Could you check a few things on this model? Use its own coordinates, in mm. Give positions to 0.01 mm unless a question says otherwise; leave off trailing zeros. Write each loop counter-clockwise with the first axis right and the second up, starting at its lowest first coordinate (ties: lowest second). Pieces come first, ordered by that corner, then holes. Notation, with made-up numbers: (57.25, 31.5) - (99.25, 31.5) arc R23 cw to (99.25, 39.5) - close; hole circle Ø8 at (58, 45). An arc over 180 degrees is marked (long way). Use one line per item in the form item = value.
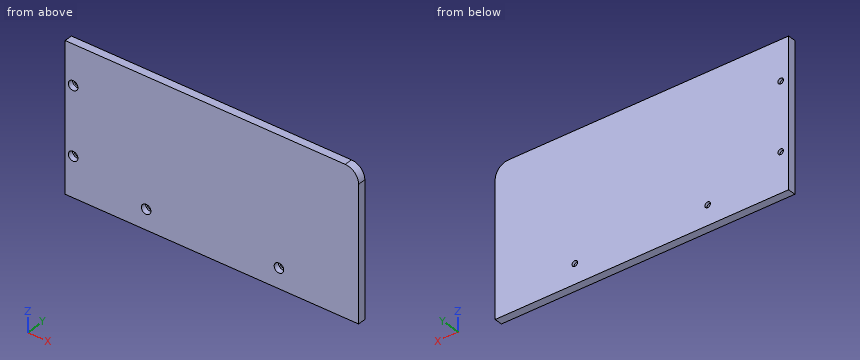
Autodesk Inventor part; units mm, degrees
ref_plane "YZ Plane" through (0, 0, 0) normal (1, 0, 0) x (0, 1, 0)
ref_plane "XZ Plane" through (0, 0, 0) normal (0, 1, 0) x (-1, 0, 0)
ref_plane "XY Plane" through (0, 0, 0) normal (0, 0, 1) x (1, 0, 0)
sketch "草图1" plane through (0, 0, 0) normal (0, 1, 0) x (-1, 0, 0)
  line L0 (110.5, 55.5) -> (-110.5, 55.5)
  line L1 (-110.5, 55.5) -> (-110.5, -55.5)
  line L2 (-110.5, -55.5) -> (110.5, -55.5)
  line L3 (110.5, -55.5) -> (110.5, 55.5)
  line L4 (0, 7.5575) -> (0, -11)
  line L5 (8.5019, 0) -> (-7, 0)
  point P0 (0, 0)
  point P1 (0, 0)
  dimension "d0" = 221
  dimension "d1" = 111
extrude "拉伸1" add sketch "草图1" along normal blind 6
fillet "圆角1" radius 10.1 1 edges at (110.5, 3, 55.5)
sketch "草图2" plane through (0, 0, 0) normal (0, -1, 0) x (1, 0, 0)
  circle A0 centre (-104.5, 25.5) radius 2.1
  circle A1 centre (-104.5, -25.5) radius 2.1
  line L0 (-110.5, -55.5) -> (-110.5, 55.5)
  line L1 (110.5, -55.5) -> (-110.5, -55.5)
  line L2 (-110.5, 55.5) -> (100.4, 55.5)
  point P0 (0, 0)
  dimension "d5" = 4.2
  dimension "d6" = 4.2
  dimension "d7" = 6
  dimension "d8" = 6
  dimension "d9" = 30
  dimension "d10" = 30
extrude "拉伸2" cut sketch "草图2" against normal blind 6
sketch "草图3" plane through (0, 0, 0) normal (0, -1, 0) x (1, 0, 0)
  circle A0 centre (-104.5, 25.5) radius 2.1
  circle A1 centre (-104.5, 25.5) radius 3.6
  circle A2 centre (-104.5, -25.5) radius 2.1
  circle A3 centre (-104.5, -25.5) radius 3.6
  point P0 (0, 0)
  dimension "d13" = 7.2
  dimension "d14" = 7.2
extrude "拉伸3" cut sketch "草图3" against normal blind 4
sketch "草图4" plane through (0, 0, 0) normal (0, -1, 0) x (1, 0, 0)
  circle A0 centre (-49.5, -40.5) radius 2.1
  circle A1 centre (50.5, -40.5) radius 2.1
  line L0 (110.5, -55.5) -> (-110.5, -55.5)
  line L1 (110.5, 45.4) -> (110.5, -55.5)
  point P0 (0, 0)
  dimension "d17" = 4.2
  dimension "d18" = 4.2
  dimension "d19" = 15
  dimension "d20" = 15
  dimension "d21" = 60
  dimension "d22" = 100
extrude "拉伸4" cut sketch "草图4" against normal blind 10
sketch "草图5" plane through (0, 0, 0) normal (0, -1, 0) x (1, 0, 0)
  circle A0 centre (-49.5, -40.5) radius 2.1
  circle A1 centre (-49.5, -40.5) radius 3.6
  circle A2 centre (50.5, -40.5) radius 2.1
  circle A3 centre (50.5, -40.5) radius 3.6
  point P0 (0, 0)
  dimension "d25" = 7.2
  dimension "d26" = 7.2
extrude "拉伸5" cut sketch "草图5" against normal blind 4 contours A0 | A1 | A2 | A3
properties part number "底板_B"
1. If I drill on line 1 (Z direction, x = -49.5, y = 5.4); line 2 (X direction, y = 3.1, z = 24), over which ranges is the centre line in solid material (lowest first)? Write a range as from..to.
Response values:
line_1 = -55.5..-42.6, -38.4..55.5
line_2 = -110.5..-107.77, -101.23..110.5
2. Imagine slicing it at B-B, the plane z = 25.5. List the corners of the cut face in (x, y) for me, and give its area (3 significant figures).
Response values:
outline = (-110.5, 0) - (-108.1, 0) - (-108.1, 4) - (-106.6, 4) - (-106.6, 6) - (-110.5, 6) - close; (-102.4, 4) - (-100.9, 4) - (-100.9, 0) - (110.5, 0) - (110.5, 6) - (-102.4, 6) - close
area = 1,290 mm²
3. Imagine slicing it at A-A, the plane x = -49.5. List the corners of the cut face in (y, z) for me.
Response values:
outline = (0, -55.5) - (6, -55.5) - (6, -42.6) - (4, -42.6) - (4, -44.1) - (0, -44.1) - close; (0, -36.9) - (4, -36.9) - (4, -38.4) - (6, -38.4) - (6, 55.5) - (0, 55.5) - close
4. Imagine slicing it at D-D, the plane x = -104.5. List the corners of the cut face in (y, z) for me, and give its area (3 significant figures).
Response values:
outline = (0, -55.5) - (6, -55.5) - (6, -27.6) - (4, -27.6) - (4, -29.1) - (0, -29.1) - close; (0, -21.9) - (4, -21.9) - (4, -23.4) - (6, -23.4) - (6, 23.4) - (4, 23.4) - (4, 21.9) - (0, 21.9) - close; (0, 29.1) - (4, 29.1) - (4, 27.6) - (6, 27.6) - (6, 55.5) - (0, 55.5) - close
area = 592 mm²
5. Imagine slicing it at C-C, the plane z = -40.5. List the corners of the cut face in (x, y) for me, and give its area (3 significant figures).
Response values:
outline = (-110.5, 0) - (-53.1, 0) - (-53.1, 4) - (-51.6, 4) - (-51.6, 6) - (-110.5, 6) - close; (-47.4, 4) - (-45.9, 4) - (-45.9, 0) - (46.9, 0) - (46.9, 4) - (48.4, 4) - (48.4, 6) - (-47.4, 6) - close; (52.6, 4) - (54.1, 4) - (54.1, 0) - (110.5, 0) - (110.5, 6) - (52.6, 6) - close
area = 1,250 mm²
6. For pin 1 (6.5 mm diameter, centred on x = -49.5, z = -40.5, fed in from -Y); pin 2 (2.5 mm diameter, centred on x = -104.5, z = -25.5, fed in from -Y), each with a flat end and sliding along its axis, tell me the tip position at first contact or that it passes through.
Response values:
pin_1 = 4
pin_2 = through
